from build123d import *

# Parameters (mm, degrees)
F0_W     = 125.1782737672
F0_H     = 104.6107336879
F1_DEPTH = 2
F2_R     = 0.99999
F3_R     = 0.99999
F4_R     = 0.99999
F5_R     = 0.99999
F6_R     = 0.99999
F7_R     = 0.9999


# Not quite as in the source:
# - a fillet or chamfer is up to 0.001 mm smaller than in the source, because OpenCascade refuses the exact size


with BuildPart() as f1:
    # F0 (on Top) → F1 (new body)
    with BuildSketch(Plane.XY):
        with Locations((2.8369072825, -2.482291311)):
            Rectangle(F0_W, F0_H)
        Polygon((39.3484285011, 22.7178257873), (39.3484285011, -22.7178257873), (0, -45.4356515746), (-39.3484285011, -22.7178257873), (-39.3484285011, 22.7178257873), (0, 45.4356515746), align=None, mode=Mode.SUBTRACT)
    extrude(amount=F1_DEPTH)

    # F2 (radius 1 in the source; OpenCascade refuses exactly that, so slightly less here)
    f2_edges = [f1.edges().sort_by_distance(p)[0] for p in [
        (-19.674214, -34.076739, 2),
        (-19.674214, -34.076739, 0),
    ]]
    fillet(f2_edges, radius=F2_R)

    # F3 (radius 1 in the source; OpenCascade refuses exactly that, so slightly less here)
    f3_edges = [f1.edges().sort_by_distance(p)[0] for p in [
        (-39.348429, 0, 2),
        (-39.348429, 0, 0),
    ]]
    fillet(f3_edges, radius=F3_R)

    # F4 (radius 1 in the source; OpenCascade refuses exactly that, so slightly less here)
    f4_edges = [f1.edges().sort_by_distance(p)[0] for p in [
        (19.674214, -34.076739, 2),
        (19.674214, -34.076739, 0),
    ]]
    fillet(f4_edges, radius=F4_R)

    # F5 (radius 1 in the source; OpenCascade refuses exactly that, so slightly less here)
    f5_edges = [f1.edges().sort_by_distance(p)[0] for p in [
        (39.348429, 0, 2),
        (39.348429, 0, 0),
    ]]
    fillet(f5_edges, radius=F5_R)

    # F6 (radius 1 in the source; OpenCascade refuses exactly that, so slightly less here)
    f6_edges = [f1.edges().sort_by_distance(p)[0] for p in [
        (-19.674214, 34.076739, 2),
        (-19.674214, 34.076739, 0),
    ]]
    fillet(f6_edges, radius=F6_R)

    # F7 (radius 1 in the source; OpenCascade refuses exactly that, so slightly less here)
    f7_edges = [f1.edges().sort_by_distance(p)[0] for p in [
        (19.674214, 34.076739, 2),
        (19.674214, 34.076739, 0),
    ]]
    fillet(f7_edges, radius=F7_R)


solid = f1.part
Can you work these out from the model? Positions are in its coordinate system, mm. A direction names the side the tool comes from. Coordinates: 2 decimals unless noted, no trailing zeros. Loops run counter-clockwise (first coordinate to the right, second up) from the corner with the lowest first, then second, coordinate; pieces in that order, holes last. Notation, with made-up numbers: (12, -33) - (32, -33) arc R19 ccw to (32, -12) - close; hole circle Ø4 at (68, -20.5). An arc over 180 degrees is marked (long way). Answer as a JSON object with one key per item and string values. Group by question number.
Item 1: On a 3-axis mill with a long thin cutter (end or side, diameter ignored), from which of +Z, -Z, +X, -X, +Y, -Y can I reach the whole of each face in a straight line? I mean faces 1 (the face through (44, -2, 2)), 2 (the face through (20.107, -34.174, 0.285)), 3 (the face through (19.542, 34.5, 1.715)). Say none if no direction works.
Item 2: If we section it at B-B (z = 1.4): List the corners of the cut face in (x, y) for me, plus the area to 3 significant figures.
Item 3: If I drill on L1, parallel to X at y = 1.5, z = 0.9; L2, parallel to Y at x = 10.5, z = 1.05; L3, parallel to Y at x = -23.5, z = 0.15, over which ranges is the centre line in solid material (lowest first)? Write a range as from..to.
Item 4: If we mould it in two halves opening along Y, with no side actions, what happens to faces 4 (the face through (-20.107, 34.174, 1.715)), 5 (the face through (44, -2, 0)), 6 (the face through (-20.1, -34.16, 1.7))? For each: released by +Y, released by -Y, zero draft, split by the parting line, or undercut.
Returned:
{
 "1": {"face 1": "+Z, +X, -X, +Y, -Y", "face 2": "-Z", "face 3": "+Z"},
 "2": {"outline": "(-59.75, -54.79) - (65.43, -54.79) - (65.43, 49.82) - (-59.75, 49.82) - close; hole (-39.43, -22.77) - (0, -45.53) - (39.43, -22.77) - (39.43, 22.77) - (0, 45.53) - (-39.43, 22.77) - close", "area": "7,710 mm²"},
 "3": {"L1": "x = -59.75..-39.35, 39.35..65.43", "L2": "y = -54.79..-39.37, 39.37..49.82", "L3": "y = -54.79..-32.41, 32.41..49.82"},
 "4": {"face 4": "undercut", "face 5": "zero draft", "face 6": "undercut"}
}
